For this review, take the finished solid that the model builds, in its own axes (mm). Round coordinates to 2 decimals unless told otherwise and drop trailing zeros. Order: outer loops, then holes, each group sorted by start corner. A loop starts at its lowest first (then second) coordinate and runs counter-clockwise, first axis right, second up. Notation, with made-up numbers: (77.5, -13.5) - (88.5, -13.5) arc R25 cw to (88.5, 2.5) - close; hole circle Ø3 at (49.5, 75). An arc over 180 degrees is marked (long way). Write each question's results on one line, items separated by ' | '. Start each with the question number.
(1) Take a section at A-A, the plane z = 0. Give the boundary of the cut face in (x, y), plus the area to 3 significant figures.
(2) Take a section at C-C, the plane x = -66.7. Give the boundary of the cut face in (y, z), plus the area to 3 significant figures.
(3) Insertion check: pin 1 Ø2 at (x, y) = (-64.5, 10.5) entering from -Z; pin 2 Ø1.5 at (x, z) = (-65, 3.5) entering from +Y. Each pin has a flat end and moves straight along its axis. Give the tip position at first contact, or say it passes through.
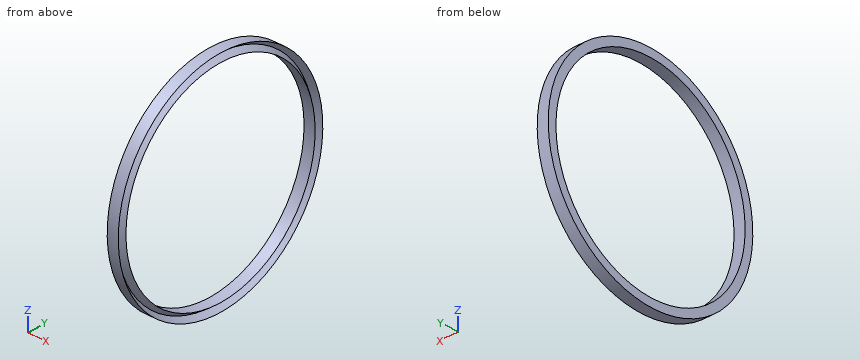
```python
from build123d import *


with BuildPart() as part:
    # Sketch1 → Revolve-Thin4 (revolve)
    with BuildSketch(Plane.XY, mode=Mode.PRIVATE) as revolve_thin4_sk:
        Polygon((-65.831423575, -38.5), (-63.830090242, -36.999), (-67.834090242, -36.999), (-67.834090242, -40.001), (-63.830090242, -40.001), align=None)
        Polygon((-65.833090242, -38.5), (-63.833090242, -37), (-67.833090242, -37), (-67.833090242, -40), (-63.833090242, -40), align=None, mode=Mode.SUBTRACT)
    revolve(revolve_thin4_sk.sketch.rotate(Axis((-81.578167515, 0, 0), (1, 0, 0)), 270), axis=Axis((-81.578167515, 0, 0), (1, 0, 0)))


solid = part.part
```
Results below:
1) outline: (-67.83, -40) - (-63.83, -40) - (-65.83, -38.5) - (-63.83, -37) - (-67.83, -37) - close; (-67.83, 37) - (-63.83, 37) - (-65.83, 38.5) - (-63.83, 40) - (-67.83, 40) - close; hole (-67.83, -40) - (-63.83, -40) - (-65.83, -38.5) - (-63.83, -37) - (-67.83, -37) - close; hole (-67.83, 37) - (-63.83, 37) - (-65.83, 38.5) - (-63.83, 40) - (-67.83, 40) - close | area: 0.0320 mm^2
2) outline: circle Ø80 at (0, 0); circle Ø74 at (0, 0); hole circle Ø80 at (0, 0); hole circle Ø74 at (0, 0) | area: 0.484 mm^2
3) pin 1: stops at z = -38.86 | pin 2: stops at y = 39.91
